from build123d import *

# Parameters (mm, degrees)
BOSS_EXTRUDE1_DEPTH = 33
SKETCH1_3_R         = 30
BOSS_EXTRUDE2_DEPTH = 40
FILLET1_R           = 22
RIB1_REACH          = 115.829
SKETCH2_WALL_W      = 306.068234896
SKETCH2_WALL_H      = 12
FILLET2_R           = 12
SKETCH3_R           = 6
CUT_EXTRUDE1_DEPTH  = 12
CUT_EXTRUDE2_START  = -12
SKETCH4_R           = 6
CUT_EXTRUDE2_DEPTH  = 12
SKETCH5_R           = 18
CUT_EXTRUDE3_DEPTH  = 80


with BuildPart() as part:
    # Sketch1 → Boss-Extrude1 (new, symmetric)
    with BuildSketch(Plane.YZ):
        with BuildLine():
            Line((-96, -24), (-96, -34))
            Line((-96, -34), (96, -34))
            Line((96, -34), (96, -24))
            Line((96, -24), (101, -24))
            Line((101, -24), (101, -16))
            Line((101, -16), (96, -16))
            Line((96, -16), (96, 12))
            Line((96, 12), (84, 12))
            Line((84, 12), (84, -22))
            Line((84, -22), (20.396078054, -22))
            ThreePointArc((20.396078054, -22), (0, -30), (-20.396078054, -22))
            Line((-20.396078054, -22), (-84, -22))
            Line((-84, -22), (-84, 12))
            Line((-84, 12), (-96, 12))
            Line((-96, 12), (-96, -16))
            Line((-96, -16), (-101, -16))
            Line((-101, -16), (-101, -24))
            Line((-101, -24), (-96, -24))
        make_face()
    extrude(amount=BOSS_EXTRUDE1_DEPTH, both=True)

    # Sketch1<3> → Boss-Extrude2 (add, symmetric)
    with BuildSketch(Plane.YZ):
        with Locations(Location((0, 0, 0), (0, 0, 270))):
            Circle(SKETCH1_3_R)
    extrude(amount=BOSS_EXTRUDE2_DEPTH, both=True)

    # Fillet1
    fillet1_edges = [part.edges().sort_by_distance(p)[0] for p in [
        (0, 20.396078054, -22),
        (0, -20.396078054, -22),
    ]]
    fillet(fillet1_edges, radius=FILLET1_R)

    # Sketch2 wall → Rib1 (add, up to next)
    with BuildSketch(Plane(origin=(0, -46.695244813, 20.246216205), x_dir=(0, 0.97642883454, 0.215839595718), z_dir=(0, -0.215839595718, 0.97642883454)), mode=Mode.PRIVATE) as rib1_sk1:
        Rectangle(SKETCH2_WALL_W, SKETCH2_WALL_H)
    rib1_tool1 = extrude(rib1_sk1.sketch, amount=-RIB1_REACH, mode=Mode.PRIVATE) - part.part
    rib1 = rib1_tool1.solids().sort_by_distance((0, -46.695244813, 20.246216205))[0]
    add(rib1)

    # Mirror1: Rib1 across plane
    add(rib1.mirror(Plane.ZX))

    # Fillet2
    fillet2_edges = [part.edges().sort_by_distance(p)[0] for p in [
        (-33, 90, 12),
        (33, -90, 12),
        (-33, -90, 12),
        (33, 90, 12),
    ]]
    fillet(fillet2_edges, radius=FILLET2_R)

    # Sketch3 → Cut-Extrude1 (cut)
    with BuildSketch(Plane(origin=(0, 96, 0), x_dir=(-1, 0, 0), z_dir=(0, 1, 0))):
        with Locations(Location((-21, 0, 0), (0, 0, 90))):
            Circle(SKETCH3_R)
        with Locations(Location((21, 0, 0), (0, 0, 90))):
            Circle(SKETCH3_R)
    extrude(amount=-CUT_EXTRUDE1_DEPTH, mode=Mode.SUBTRACT)

    # Sketch4 → Cut-Extrude2 (cut)
    with BuildSketch(Plane.XZ.offset(96).offset(CUT_EXTRUDE2_START)):
        with Locations(Location((-21, 0, 0), (0, 0, 90))):
            Circle(SKETCH4_R)
        with Locations(Location((21, 0, 0), (0, 0, 90))):
            Circle(SKETCH4_R)
    extrude(amount=CUT_EXTRUDE2_DEPTH, mode=Mode.SUBTRACT)

    # Sketch5 → Cut-Extrude3 (cut)
    with BuildSketch(Plane.YZ.offset(40)):
        with Locations(Location((0, 0, 0), (0, 0, 270))):
            Circle(SKETCH5_R)
    extrude(amount=-CUT_EXTRUDE3_DEPTH, mode=Mode.SUBTRACT)


solid = part.part
The listing builds one solid part. Answer for the finished solid, in the listing's coordinates (mm). A direction names the side the tool comes from. Round coordinates to 2 decimals unless told otherwise and drop trailing zeros. Loops run counter-clockwise (first coordinate to the right, second up) from the corner with the lowest first, then second, coordinate; pieces in that order, holes last. Notation, with made-up numbers: M 23.25,21 L 67.25,21 A28 ccw 67.25,60 Z; hole C -21.75,48.25 d7. An arc over 180 degrees is marked long. Return JSON: item names as keys, results as strings.
Q1. Find the intervals of material crossed by line 1 along Y through (x, z) = (9, 5); line 2 along Y through (x, z) = (-21.5, -19); line 3 along Y through (x, z) = (9, 10), in increasing order. Write a range as from..to.
Results list:
{"line 1": "y = -96..-84, -29.58..-17.29, 17.29..29.58, 84..96", "line 2": "y = -101..-84, -40.91..40.91, 84..101", "line 3": "y = -96..-84, -28.28..-14.97, 14.97..28.28, 84..96"}
Q2. Find section B-B, the plane y = 86. Determine the outline of the cut face in (x, z).
Results list:
{"outline": "M -33,-34 L 33,-34 L 33,0 A12 ccw 21,12 L -21,12 A12 ccw -33,0 Z; hole C -21,0 d12; hole C 21,0 d12"}
Q3. Each of these flat-tipped pins is pushed along its axis until it touches: pin 1 Ø5 at (x, y) = (23.5, -25.5) entering from +Z; pin 2 Ø8 at (x, y) = (19.5, -62.5) entering from +Z; pin 3 Ø10 at (x, z) = (-9.5, 7.5) entering from +Y. Where does it stop, or does it pass through?
Results list:
{"pin 1": "stops at z = 19.26", "pin 2": "stops at z = -22", "pin 3": "stops at y = 96"}
Q4. Find section A-A, the plane x = -24.5. State how many separate pieces and enclosed holes the cut face has, plus the area to 3 significant figures.
Results list:
{"separate pieces": "3", "enclosed holes": "1", "area": "4,880 mm2"}
Q5. The mould has two halves that part along Z. Classify faces 5 (the face through (-6, -56, -2)), 6 (the face through (-22.802, -89.916, 5.723)), 7 (the face through (20, 68, -22)): released by +Z, released by -Z, zero draft, split by the parting line, or undercut.
Results list:
{"face 5": "zero draft", "face 6": "undercut", "face 7": "released by +Z"}
Q6. Find section D-D, the plane x = 0.5. Determine the outline of the cut face in (y, z), plus the area to 3 significant figures.
Results list:
{"outline": "M -101,-24 L -96,-24 L -96,-34 L 96,-34 L 96,-24 L 101,-24 L 101,-16 L 96,-16 L 96,12 L 84,12 L 9.39,28.49 A30 ccw -9.39,28.49 L -84,12 L -96,12 L -96,-16 L -101,-16 Z; hole C 0,0 d36", "area": "9,450 mm2"}
Q7. Which of the six approach directions +Z, -Z, +X, -X, +Y, -Y give full straight-line access (tool end or side, diameter ignored) to faces 1 (the face through (-15.05, 90.08, -0.78)), 2 (the face through (-19, 84, -9)), 3 (the face through (0, -90, 12)), 4 (the face through (19.69, -36.27, -15.38))?
Results list:
{"face 1": "+Y", "face 2": "+Z, -X", "face 3": "+Z, +X, -X, -Y", "face 4": "+Z, +X"}
